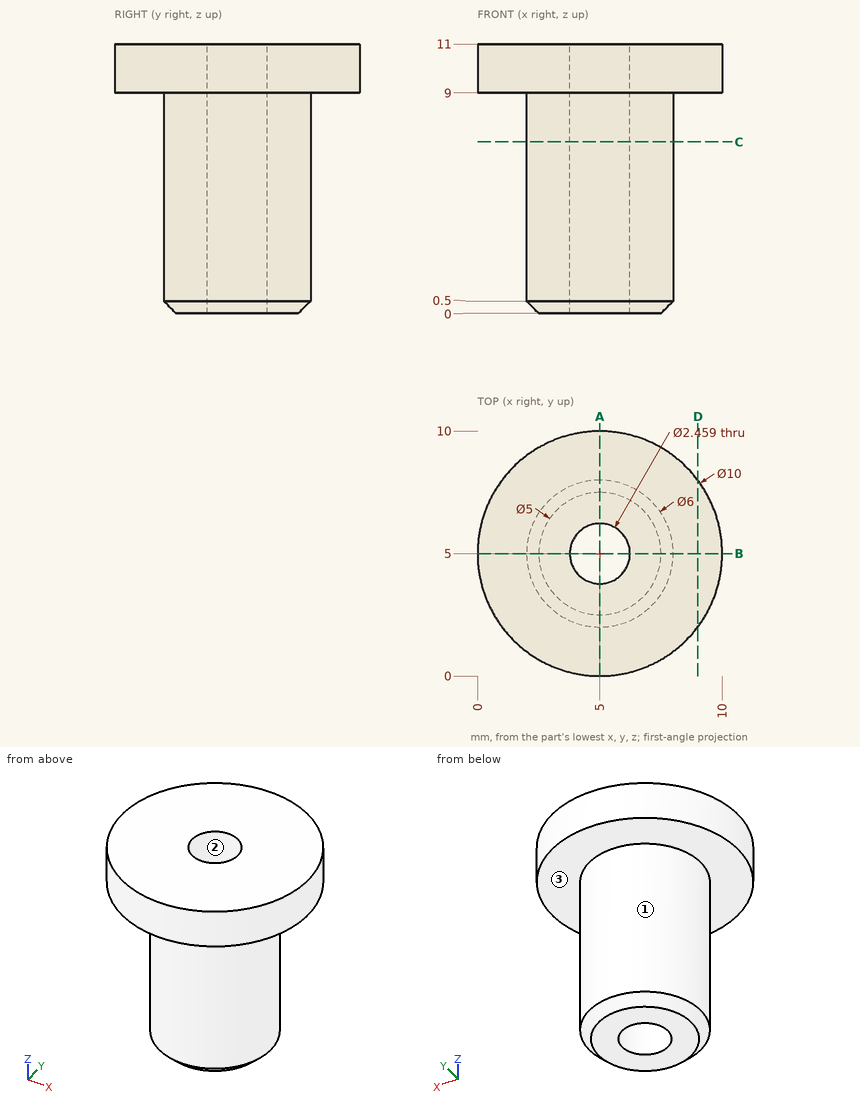
Print and shaded views of the part. All mm, measured from the part's lowest x, y and z. Coordinates: 2 decimals unless noted, no trailing zeros. Order: outer loops, then holes, each group sorted by start corner. A loop starts at its lowest first (then second) coordinate and runs counter-clockwise, first axis right, second up. Notation, with made-up numbers: (35, 30.5) -> (53, 30.5) arc R29 ccw to (53, 52.5) -> close; hole circle Ø1 at (-18.5, 88.5). An arc over 180 degrees is marked (long way). Use one line per item in the form item = value. Start each with the question number.
1) Pull direction X, two halves, no side cores. Call the marked faces 1, 2 and 3: +X half, -X half, draft (parallel to the pull), parting line (faces both ways), or undercut.
2) Band-saw the part on D-D on x = 9. Give the cut face in (y, z).
3) Drill centre lines: L1, parallel to X at y = 5, z = 7; L2, parallel to Z at x = 6.25, y = 9.5. Where is each one in solid material? Low to high. Write a range as [from, to].
4) Band-saw the part on C-C on z = 7. Give the cut face in (x, y).
5) Drop flat-ended pins along their axis: pin 1 (3 mm diameter, centred on x = 7, z = 5, fed in from -Y); pin 2 (5 mm diameter, centred on y = 4.5, z = 4, fed in from -X); pin 3 (1.5 mm diameter, centred on x = 5, y = 5, fed in from +Z); pin 4 (6 mm diameter, centred on x = 7.5, z = 6.5, fed in from -Y). Give the stop position or say it passes through.
6) Band-saw the part on A-A on x = 5. Give the cut face in (y, z), then the cut area to 3 significant figures.
Entries:
q1.face_1 = parting line
q1.face_2 = undercut
q1.face_3 = draft
q2.outline = (2, 9) -> (8, 9) -> (8, 11) -> (2, 11) -> close
q3.L1 = [2, 3.77], [6.23, 8]
q3.L2 = [9, 11]
q4.outline = circle Ø6 at (5, 5); hole circle Ø2.46 at (5, 5)
q5.pin_1 = 2.04
q5.pin_2 = 2
q5.pin_3 = through
q5.pin_4 = 0.07
q6.outline = (0, 9) -> (2, 9) -> (2, 0.5) -> (2.5, 0) -> (3.77, 0) -> (3.77, 11) -> (0, 11) -> close; (6.23, 0) -> (7.5, 0) -> (8, 0.5) -> (8, 9) -> (10, 9) -> (10, 11) -> (6.23, 11) -> close
q6.area = 46.7 mm2
